Design review of the part built by this model. Coordinates are the model's own, in mm. Face numbers are marked on the shaded views. A direction names the side the tool comes from. Coordinates: 2 decimals unless noted, no trailing zeros. Write each loop counter-clockwise with the first axis right and the second up, starting at its lowest first coordinate (ties: lowest second). Pieces come first, ordered by that corner, then holes.
Q1. For the marked faces 5 and 6, list the 3-axis set-ups (+Z, -Z, +X, -X, +Y, -Y) from which the entire face can be reached by the end or side of a thin tool; tool diameter is ignored.
Q2. Take a section at C-C, the plane x = 2. Write out the cut boundary in (y, z).
Q3. Take a section at A-A, the plane x = 0. Write out the cut boundary in (y, z), plus the area to 3 significant figures.
Q4. For L1, parallel to Y at x = 0, z = 1.1; L2, parallel to Y at x = 0, z = 2.6; L3, parallel to Z at x = -0.5, y = 2.5, list the stretches that pass through material, from the lowest coordinate up.
Q5. The part is to be moulded in two halves that separate along Y. For the marked faces 1, 2, 3 and 4, say which applies: released by +Y, released by -Y, zero draft, split by the parting line, or undercut.
Q6. For pin 1 Ø1.8 at (x, y) = (0, 0) entering from -Z, flat-tipped, find the tip position at first contact; note if it passes through.
from build123d import *

# Parameters (mm, degrees)
BOSS_EXTRUDE1_DEPTH = 4
SKETCH2_R           = 1.5
CUT_EXTRUDE1_DEPTH  = 4
SKETCH3_R           = 3
CUT_EXTRUDE2_DEPTH  = 2


with BuildPart() as part:
    # Sketch1 → Boss-Extrude1 (new body)
    with BuildSketch(Plane.XY):
        with BuildLine():
            Line((-3.399881961, 2.8), (-3.399881961, -2.8))
            add(Edge.make_bspline(
                [(-3.399881961, -2.8), (-3.399881961, -2.953071187), (-3.271882834, -3.271984466), (-2.952966029, -3.4), (-2.799893385, -3.4)],
                knots=[-1.570796327, -1.570796327, -1.570796327, -1.570796327, -0.785398163, 0, 0, 0, 0], degree=3))
            Line((-2.799893385, -3.4), (2.799893385, -3.4))
            add(Edge.make_bspline(
                [(2.799893385, -3.4), (2.952966029, -3.4), (3.271882834, -3.271984466), (3.399881961, -2.953071187), (3.399881961, -2.8)],
                knots=[0, 0, 0, 0, 0.785398163, 1.570796327, 1.570796327, 1.570796327, 1.570796327], degree=3))
            Line((3.399881961, -2.8), (3.399881961, 2.8))
            add(Edge.make_bspline(
                [(3.399881961, 2.8), (3.399881961, 2.953071187), (3.271882834, 3.271984466), (2.952966029, 3.4), (2.799893385, 3.4)],
                knots=[1.570796327, 1.570796327, 1.570796327, 1.570796327, 2.35619449, 3.141592654, 3.141592654, 3.141592654, 3.141592654], degree=3))
            Line((2.799893385, 3.4), (-2.799893385, 3.4))
            add(Edge.make_bspline(
                [(-2.799893385, 3.4), (-2.952966029, 3.4), (-3.271882834, 3.271984466), (-3.399881961, 2.953071187), (-3.399881961, 2.8)],
                knots=[-3.141592654, -3.141592654, -3.141592654, -3.141592654, -2.35619449, -1.570796327, -1.570796327, -1.570796327, -1.570796327], degree=3))
        make_face()
    extrude(amount=BOSS_EXTRUDE1_DEPTH)

    # Sketch2 → Cut-Extrude1 (cut)
    with BuildSketch(Plane.XY.offset(4)):
        Circle(SKETCH2_R)
    extrude(amount=-CUT_EXTRUDE1_DEPTH, mode=Mode.SUBTRACT)

    # Sketch3 → Cut-Extrude2 (cut)
    with BuildSketch(Plane(origin=(0, 0, 0), x_dir=(-1, 0, 0), z_dir=(0, 0, -1))):
        Circle(SKETCH3_R)
    extrude(amount=-CUT_EXTRUDE2_DEPTH, mode=Mode.SUBTRACT)


solid = part.part
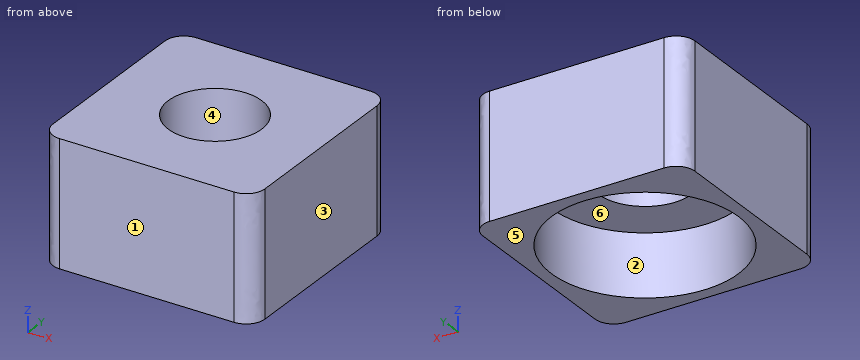
Responses:
1. face 5: -Z, +X, -X, +Y, -Y
1. face 6: -Z
2. outline: (-3.4, 0) - (-2.24, 0) - (-2.24, 2) - (2.24, 2) - (2.24, 0) - (3.4, 0) - (3.4, 4) - (-3.4, 4) - close
3. outline: (-3.4, 0) - (-3, 0) - (-3, 2) - (-1.5, 2) - (-1.5, 4) - (-3.4, 4) - close; (1.5, 2) - (3, 2) - (3, 0) - (3.4, 0) - (3.4, 4) - (1.5, 4) - close
3. area: 9.20 mm2
4. L1: y = -3.4 to -3, 3 to 3.4
4. L2: y = -3.4 to -1.5, 1.5 to 3.4
4. L3: z = 2 to 4
5. face 1: released by -Y
5. face 2: undercut
5. face 3: zero draft
5. face 4: undercut
6. pin 1: passes through
